Verification items for the finished model (mm, model axes). A direction names the side the tool comes from. Round coordinates to 2 decimals unless told otherwise and drop trailing zeros. Write each loop counter-clockwise with the first axis right and the second up, starting at its lowest first coordinate (ties: lowest second). Pieces come first, ordered by that corner, then holes.
from build123d import *

# Parameters (mm, degrees)
F0_R          = 60
F0_R_2        = 20
F1_DEPTH      = 1000
F3_R          = 20
F4_DEPTH      = 100
F4_DEPTH_BACK = 7
F6_R          = 20
F7_DEPTH      = 100
F7_DEPTH_BACK = 7


with BuildPart() as f1:
    # F0 (on Front) → F1 (new body)
    with BuildSketch(Plane.XZ):
        Circle(F0_R)
        Circle(F0_R_2, mode=Mode.SUBTRACT)
    extrude(amount=F1_DEPTH)

    # F3 (on offset) → F4 (join, two sides)
    with BuildSketch(Plane.XY.offset(60)) as f4_sk:
        with Locations((0, -20)):
            Circle(F3_R)
    extrude(amount=F4_DEPTH)
    extrude(f4_sk.sketch, amount=-F4_DEPTH_BACK)

    # F6 (on offset) → F7 (join, two sides)
    with BuildSketch(Plane.XY.offset(-60)) as f7_sk:
        with Locations((0, -980)):
            Circle(F6_R)
    extrude(amount=-F7_DEPTH)
    extrude(f7_sk.sketch, amount=F7_DEPTH_BACK)


solid = f1.part
Q1. Sectioned sample at B-B (y = -980). Enter the section's corners in (x, z), plus the area to 3 significant figures.
Recorded:
outline: (-20, -160) - (20, -160) - (20, -56.57) arc R60 ccw (long way) to (-20, -56.57) - close; hole circle Ø40 at (0, 0)
area: 14,100 mm2
Q2. Sectioned sample at A-A (z = 0). Enter the section's corners in (x, y).
Recorded:
outline: (-60, -1000) - (-20, -1000) - (-20, 0) - (-60, 0) - close; (20, -1000) - (60, -1000) - (60, 0) - (20, 0) - close
Q3. Tool access check on faces 4 (the cylindrical face through (-2.6, -960.17, -109.01)), 5 (the flat face through (0, -20, 160)). Record the directions out of +Z, -Z, +X, -X, +Y, -Y that give a thin tool (end or side, any length) a straight path to the whole face; none if there is none.
Recorded:
face 4: -Z
face 5: +Z, +X, -X, +Y, -Y
Q4. Sectioned sample at D-D (x = -39.5). Enter the section's corners in (y, z), plus the area to 3 significant figures.
Recorded:
outline: (-1000, -45.16) - (0, -45.16) - (0, 45.16) - (-1000, 45.16) - close
area: 90,300 mm2
Q5. Release check for a two-part mould opening along X. For faces 1 (the cylindrical face through (-59.94, -493, 2.64)), 2 (the flat face through (0, -980, -160)), 3 (the cylindrical face through (-4.336, -493, -19.524)) record: released by +X, released by -X, zero draft, split by the parting line, or undercut.
Recorded:
face 1: split by the parting line
face 2: zero draft
face 3: undercut
Q6. Material ranges on line 1 along Z through (x, y) = (0, -751); line 2 along Z through (x, y) = (-3.5, -162.5); line 3 along X through (y, z) = (-237, -10), recorded low to high.
Recorded:
line 1: z = -60 to -20, 20 to 60
line 2: z = -59.9 to -19.69, 19.69 to 59.9
line 3: x = -59.16 to -17.32, 17.32 to 59.16
Q7. Depth check by flat-ended pin: P1, Ø5, axis at x = 15.5, y = -634.5, coming from the +Z side; P2, Ø1.5, axis at x = 0.5, y = -786, coming from the +Z side; P3, Ø8, axis at x = 36, y = -560, coming from the +Z side. Enter the tip coordinate at first touch or a pass-through.
Recorded:
P1: stops at z = 58.57
P2: stops at z = 60
P3: stops at z = 50.75
Q8. Sectioned sample at C-C (z = 108.5). Enter the section's corners in (x, y), plus the area to 3 significant figures.
Recorded:
outline: circle Ø40 at (0, -20)
area: 1,260 mm2
